Part model, mm, in its own coordinate system. A direction names the side the tool comes from. Round coordinates to 2 decimals unless told otherwise and drop trailing zeros. Order: outer loops, then holes, each group sorted by start corner. A loop starts at its lowest first (then second) coordinate and runs counter-clockwise, first axis right, second up. Notation, with made-up numbers: (-7.5, -4.5) - (39.5, -4.5) arc R31 cw to (39.5, 20.5) - close; hole circle Ø11 at (-16, 88). An arc over 180 degrees is marked (long way). Return JSON: item names as keys, results as strings. Group by question number.
Item 1: Saw through at C-C on y = -22.5. List the corners of the cut face in (x, z), and give its area (3 significant figures).
Item 2: Tool access for faces 1 (the face through (0, -38, 21)), 2 (the face through (-2, -14.198, -38)), 3 (the face through (15.74, -31.16, 47.4)), 4 (the face through (2.525, -60.818, 46.089)), 5 (the face through (-16.571, -13, 16)): list every direction of +Z, -Z, +X, -X, +Y, -Y with a clear straight run to the whole face (end or side of a thin tool).
Item 3: Saw through at D-D on z = 70.5. List the corners of the cut face in (x, y), and give its area (3 significant figures).
Item 4: Probe probe 1 along Y at (x, z) = (-3.5, -27); probe 2 along X at (y, z) = (-15, 23); probe 3 along Y at (x, z) = (14.75, 50.8). List the from-to ranges inside material, lowest first.
Item 5: Drop flat-ended pins along their axis: pin 1 (23 mm diameter, centred on y = -39.2, z = 50.8, fed in from -X); pin 2 (10 mm diameter, centred on x = -10.5, y = -26, fed in from +Z); pin 3 (5 mm diameter, centred on y = -45.5, z = 34, fed in from -X). Give the stop position or say it passes through.
Item 6: Saw through at B-B on y = -60. List the corners of the cut face in (x, z).
Item 7: Two-plate mould, pull along Z, no slides. Class faces 6 (the face through (8, -12, -35.737)), 7 (the face through (7, -49.53, 22)), 8 (the face through (-3.81, -10, -38)): released by +Z, released by -Z, zero draft, split by the parting line, or undercut.
```python
from build123d import *

# Parameters (mm, degrees)
F1_DEPTH  = 25.4
F2_W      = 15.1281697808
F2_H      = 88.9
F3_DEPTH  = 25.4
F4_R      = 6.35
F5_DEPTH  = 20.32
F7_R      = 10.16
F8_DEPTH  = 2.54
F6_R      = 10.16
F9_DEPTH  = 2.54
F10_T     = -1.27
F11_R     = 6.35
F11_R_2   = 3.556
F12_DEPTH = 5.08
F13_R     = 5.08
F14_DEPTH = 25.4


with BuildPart() as f1:
    # F0 (on Front) → F1 (new body)
    with BuildSketch(Plane.XZ):
        Polygon((-17.8410302192, 65.8628800811), (-17.8410302192, -35.7371199189), (32.9589697808, -35.7371199189), (32.9589697808, 65.8628800811), (7.5589697808, 109.8569705933), align=None)
    extrude(amount=F1_DEPTH)

    # F2 (on face) → F3 (join)
    with BuildSketch(Plane.XZ.offset(25.4)):
        with Locations((7.5640848904, 21.4128800811)):
            Rectangle(F2_W, F2_H)
    extrude(amount=F3_DEPTH)

    # F4 (on face) → F5 (join)
    with BuildSketch(Plane.XZ.offset(50.8)):
        with Locations((7.5640848904, 49.9533750117)):
            Circle(F4_R)
        with Locations((7.5640848904, 30.7380091399)):
            Circle(F4_R)
        with Locations((7.5640848904, 11.1665166914)):
            Circle(F4_R)
        with Locations((7.5640848904, -10.9471287578)):
            Circle(F4_R)
    extrude(amount=F5_DEPTH)

    # F7 (on face) → F8 (join)
    with BuildSketch(Plane.YZ.offset(15.1281697808)):
        with Locations((-38.9532968402, 0)):
            Circle(F7_R)
        with Locations((-39.375923574, 50.8)):
            Circle(F7_R)
    extrude(amount=F8_DEPTH)

    # F6 (on face) → F9 (join)
    with BuildSketch(Plane(origin=(0, 0, 0), x_dir=(0, -1, 0), z_dir=(-1, 0, 0))):
        with Locations((39.2042249441, 50.8)):
            Circle(F6_R)
        with Locations((39.2042249441, 0)):
            Circle(F6_R)
    extrude(amount=F9_DEPTH)

    # F10
    f10_openings = [f1.faces().sort_by_distance(p)[0] for p in [
        (17.66817, -38.953297, 0),
        (17.66817, -39.375924, 50.8),
        (-2.54, -39.204225, 50.8),
        (-2.54, -39.204225, 0),
    ]]
    offset(amount=F10_T, openings=f10_openings, kind=Kind.INTERSECTION)

    # F11 (on face) → F12 (join)
    with BuildSketch(Plane(origin=(0, 0, -35.7371199189), x_dir=(1, 0, 0), z_dir=(0, 0, -1))):
        with Locations((7.5692, 11.8115022779)):
            Circle(F11_R)
        with Locations((7.5692, 11.8115022779)):
            Circle(F11_R_2, mode=Mode.SUBTRACT)
        Polygon((0, 19.2781486231), (-12.7, 19.2781486231), (-12.7, 14.1981486231), (-8.89, 14.1981486231), (-8.89, 6.5781486231), (-3.81, 6.5781486231), (-3.81, 14.1981486231), (0, 14.1981486231), align=None)
        Polygon((27.8281697808, 19.2781486231), (15.1281697808, 19.2781486231), (15.1281697808, 14.1981486231), (18.9381697808, 14.1981486231), (18.9381697808, 6.5781486231), (24.0181697808, 6.5781486231), (24.0181697808, 14.1981486231), (27.8281697808, 14.1981486231), align=None)
    extrude(amount=F12_DEPTH)

    # F13 (on face) → F14 (join)
    with BuildSketch(Plane.XZ.offset(25.4)):
        with Locations((8.3121880889, 80.7227864861)):
            Circle(F13_R)
    extrude(amount=F14_DEPTH)


solid = f1.part
```
Filled in:
{
 "1": {"outline": "(-17.84, -35.74) - (32.96, -35.74) - (32.96, 65.86) - (7.56, 109.86) - (-17.84, 65.86) - close; hole (-16.57, -34.47) - (31.69, -34.47) - (31.69, 65.52) - (7.56, 107.32) - (-16.57, 65.52) - close", "area": "445 mm^2"},
 "2": {"face 1": "-X", "face 2": "-Z, +Y", "face 3": "+X", "face 4": "-Y", "face 5": "none"},
 "3": {"outline": "(-15.16, -25.4) - (30.28, -25.4) - (30.28, 0) - (-15.16, 0) - close; hole (-13.7, -24.13) - (28.82, -24.13) - (28.82, -1.27) - (-13.7, -1.27) - close", "area": "182 mm^2"},
 "4": {"probe 1": "y = -25.4 to -24.13, -1.27 to 0", "probe 2": "x = -17.84 to -16.57, 31.69 to 32.96", "probe 3": "y = -50.8 to -48.27, -30.49 to -24.13, -1.27 to 0"},
 "5": {"pin 1": "stops at x = -2.54", "pin 2": "stops at z = 87.18", "pin 3": "stops at x = 0"},
 "6": {"outline": "circle Ø12.7 at (7.56, -10.95); circle Ø12.7 at (7.56, 11.17); circle Ø12.7 at (7.56, 30.74); circle Ø12.7 at (7.56, 49.95); hole circle Ø10.16 at (7.56, -10.95); hole circle Ø10.16 at (7.56, 11.17); hole circle Ø10.16 at (7.56, 30.74); hole circle Ø10.16 at (7.56, 49.95)"},
 "7": {"face 6": "released by -Z", "face 7": "undercut", "face 8": "zero draft"}
}
